Check sheet for the drawn part. Datum: minimum x, y, z corner. Units: mm. Give positions to 0.01 mm unless a question says otherwise; leave off trailing zeros. Order: outer loops, then holes, each group sorted by start corner. A loop starts at its lowest first (then second) coordinate and runs counter-clockwise, first axis right, second up. Notation, with made-up numbers: (75.5, 63) -> (98.5, 63) arc R9 cw to (98.5, 76) -> close; hole circle Ø10 at (-14, 35.25). An arc over 180 degrees is marked (long way). Return JSON: item names as keys, results as strings. Group by question number.
(1) Depth check by flat-ended pin: pin 1 Ø10 at (x, y) = (48, 52) entering from -Z; pin 2 Ø8 at (x, y) = (48, 49.5) entering from -Z; pin 3 Ø5 at (y, z) = (125.5, 45.5) entering from +X. Enter the tip coordinate at first touch or a pass-through.
(2) Cross-section at B-B on z = 51.5. Enter the section's corners in (x, y).
(3) Cross-section at D-D on y = 22.5. Enter the section's corners in (x, z), then the cut area to 3 significant figures.
(4) Cross-section at C-C on y = 123. Enter the section's corners in (x, z).
(5) Release check for a two-part mould opening along X. For the marked faces 1, 2 and 3 record: pulls with the +X half, pulls with the -X half, needs draft (parallel to the pull), parting line crosses it, or undercut.
(6) Cross-section at A-A on x = 28. Enter the section's corners in (y, z), then the cut area to 3 significant figures.
(7) Thickness scan on line 1 along Z through (x, y) = (29, 87.5); line 2 along X through (y, z) = (140, 5); line 3 along Z through (x, y) = (44, 75). Record the ranges inside material, lowest first.
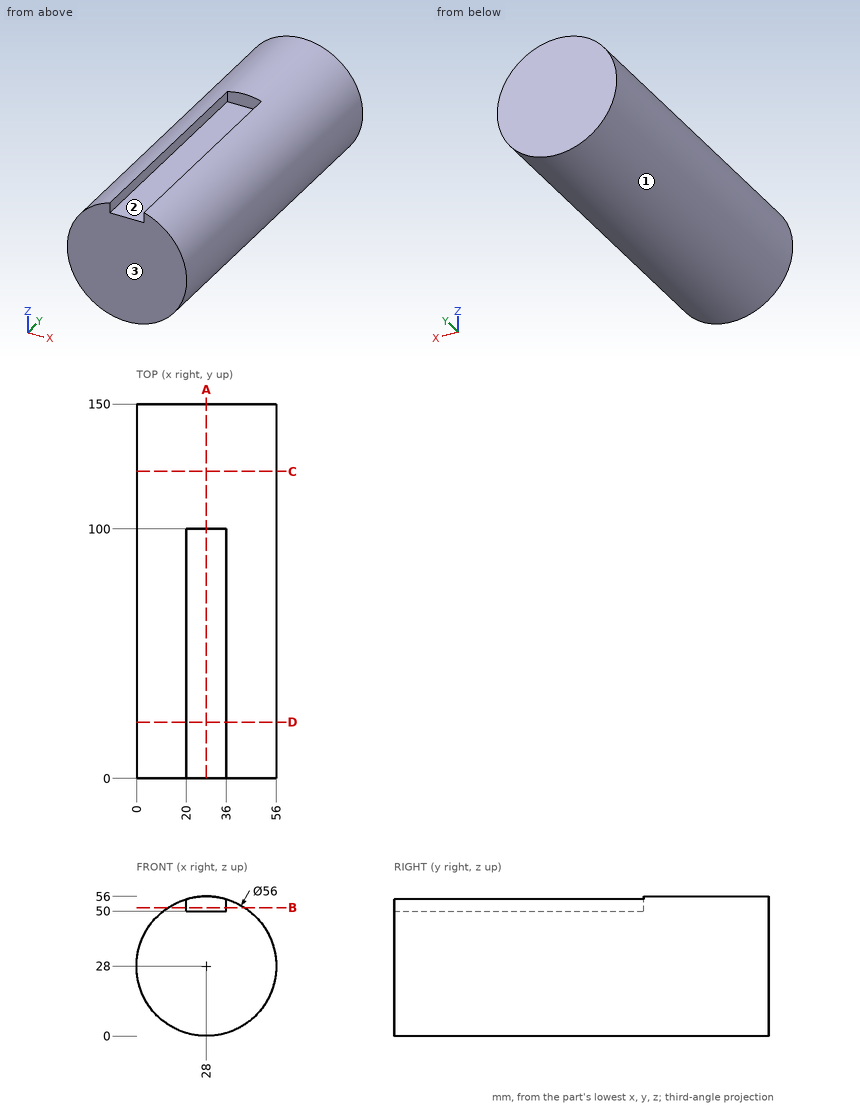
Verdict:
{
 "1": {"pin 1": "z = 4.36", "pin 2": "z = 5.02", "pin 3": "x = 51.64"},
 "2": {"outline": "(12.78, 0) -> (20, 0) -> (20, 100) -> (36, 100) -> (36, 0) -> (43.22, 0) -> (43.22, 150) -> (12.78, 150) -> close"},
 "3": {"outline": "(20, 50) -> (20, 54.83) arc R28 ccw (long way) to (36, 54.83) -> (36, 50) -> close", "area": "2,370 mm²"},
 "4": {"outline": "circle Ø56 at (28, 28)"},
 "5": {"face 1": "parting line crosses it", "face 2": "undercut", "face 3": "needs draft"},
 "6": {"outline": "(0, 0) -> (150, 0) -> (150, 56) -> (100, 56) -> (100, 50) -> (0, 50) -> close", "area": "7,800 mm²"},
 "7": {"line 1": "0.02 to 50", "line 2": "12.03 to 43.97", "line 3": "5.02 to 50.98"}
}
